Design review of the part built by this model. Coordinates are the model's own, in mm. Coordinates: 2 decimals unless noted, no trailing zeros. Loops run counter-clockwise (first coordinate to the right, second up) from the corner with the lowest first, then second, coordinate; pieces in that order, holes last. Notation, with made-up numbers: (0, 75) -> (11, 75) arc R29 ccw to (11, 106) -> close; hole circle Ø3 at (-23.5, 16). An arc over 180 degrees is marked (long way). Use a Markdown table: item, result. Add a question column.
Q1. Take a section at B-B on z = 24.5. Write out the cut boundary in (x, y).
Q2. Take a section at A-A on z = 12.5. Write out the cut boundary in (x, y).
Q3. Clearance check with flat-ended pins moving along their axes: pin 1 Ø12 at (x, y) = (35.5, -48) entering from -Z; pin 2 Ø12 at (x, y) = (50.5, -8.5) entering from -Z; pin 3 Ø8 at (x, y) = (33.5, -9) entering from +Z. State where each tip first meets the part, or that it passes through.
Q4. For probe 1 along Y at (x, z) = (1.5, 46.5); probe 2 along Z at (x, y) = (42.5, 7.5); probe 3 along Z at (x, y) = (-39.5, 31), list the stretches that pass through material, from the lowest coordinate up.
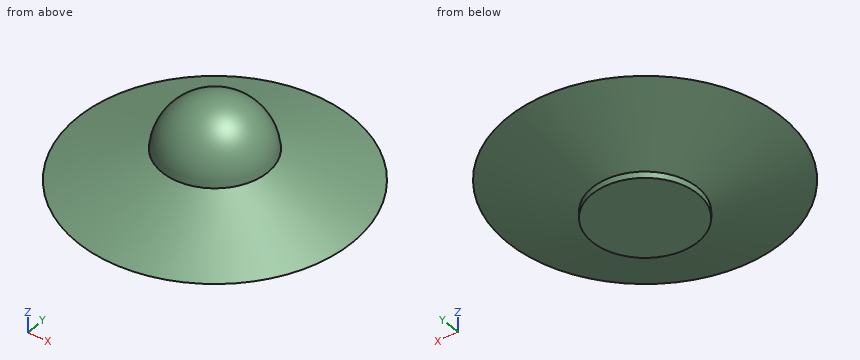
from build123d import *

# Parameters (mm, degrees)
F2_R      = 65
F3_R      = 25
F5_FACE_R = 65
F4_R      = 25
F7_DEPTH  = 23
F9_DEPTH  = 3


# Not quite as in the source:
# - a fillet or chamfer that OpenCascade refuses, or shapes differently, is made with other operations: its cross-section is extruded or revolved along the edge and cut away or added


with BuildPart() as f5:
    # F2 (on offset) → F5 section 0
    with BuildSketch(Plane.XY.offset(15)):
        Circle(F2_R)
    # F3 (on offset) → F5 section 1
    with BuildSketch(Plane.XY.offset(30)):
        Circle(F3_R)
    loft()

    # F5_face (on face) → F6 section 0
    with BuildSketch(Plane(origin=(0, 0, 15), x_dir=(1, 0, 0), z_dir=(0, 0, -1))):
        Circle(F5_FACE_R)
    # F4 (on Top) → F6 section 1
    with BuildSketch(Plane.XY):
        Circle(F4_R)
    loft()

    # F7 (add): a face of the model
    f7_faces = [f5.faces().sort_by_distance(p)[0] for p in [
        (0, 0, 30),
    ]]
    extrude(f7_faces, amount=F7_DEPTH)

    # F8: fillet of radius 25 on 1 edges, made by hand

    # F8_s1 → F8_t2 (revolve, cut)
    with BuildSketch(Plane.XZ):
        with BuildLine():
            ThreePointArc((25, 30), (17.0359533691, 46.3711730709), (0.0801284112, 53))
            Line((0.0801284112, 53), (25, 53))
            Line((25, 53), (25, 30))
        make_face()
    revolve(axis=Axis((0, 0, 53), (0, 0, 1)), mode=Mode.SUBTRACT)

    # F9 (add): a face of the model
    f9_faces = [f5.faces().sort_by_distance(p)[0] for p in [
        (0, 0, 0),
    ]]
    extrude(f9_faces, amount=F9_DEPTH)


solid = f5.part
Answer list:
| question | item | result |
|---|---|---|
| 1 | outline | circle Ø79.33 at (0, 0) |
| 2 | outline | circle Ø116.67 at (0, 0) |
| 3 | pin 1 | z = 10.76 |
| 3 | pin 2 | z = 7.58 |
| 3 | pin 3 | z = 27.87 |
| 4 | probe 1 | -16.83 to 16.83 |
| 4 | probe 2 | 6.81 to 23.19 |
| 4 | probe 3 | 9.45 to 20.55 |
